from build123d import *

# Parameters (mm, degrees)
SKETCH1_R           = 1.5875
SKETCH1_W           = 12.7
SKETCH1_H           = 6.35
SKETCH1_W_2         = 6.35
BOSS_EXTRUDE1_DEPTH = 6.35


with BuildPart() as part:
    # Sketch1 → Boss-Extrude1 (new body)
    # profile 1 of 6: a face of its own
    with BuildSketch(Plane(origin=(0, 0, 0), x_dir=(1, 0, 0), z_dir=(0, 1, 0))):
        Polygon((355.6, 19.05), (177.8, 19.05), (177.8, 0), (355.6, 0), (355.6, 6.35), (355.6, 12.7), align=None)
        with Locations(Location((196.05625, 9.525, 0), (0, 0, 270))):
            Circle(SKETCH1_R, mode=Mode.SUBTRACT)
        with Locations((298.45, 9.525)):
            Rectangle(SKETCH1_W, SKETCH1_H, mode=Mode.SUBTRACT)
    # profile 2 of 6: a face of its own
    with BuildSketch(Plane(origin=(0, 0, 0), x_dir=(1, 0, 0), z_dir=(0, 1, 0))):
        Polygon((177.8, 0), (177.8, 19.05), (0, 19.05), (0, 12.7), (0, 6.35), (0, 0), align=None)
        with Locations(Location((159.54375, 9.525, 0), (0, 0, 270))):
            Circle(SKETCH1_R, mode=Mode.SUBTRACT)
    # profile 3 of 6: a face of its own
    with BuildSketch(Plane(origin=(0, 0, 0), x_dir=(1, 0, 0), z_dir=(0, 1, 0))):
        with Locations((-3.175, 15.875)):
            Rectangle(SKETCH1_W_2, SKETCH1_H)
    # profile 4 of 6: a face of its own
    with BuildSketch(Plane(origin=(0, 0, 0), x_dir=(1, 0, 0), z_dir=(0, 1, 0))):
        with Locations((358.775, 15.875)):
            Rectangle(SKETCH1_W_2, SKETCH1_H)
    # profile 5 of 6: a face of its own
    with BuildSketch(Plane(origin=(0, 0, 0), x_dir=(1, 0, 0), z_dir=(0, 1, 0))):
        with Locations((-3.175, 3.175)):
            Rectangle(SKETCH1_W_2, SKETCH1_H)
    # profile 6 of 6: a face of its own
    with BuildSketch(Plane(origin=(0, 0, 0), x_dir=(1, 0, 0), z_dir=(0, 1, 0))):
        with Locations((358.775, 3.175)):
            Rectangle(SKETCH1_W_2, SKETCH1_H)
    extrude(amount=BOSS_EXTRUDE1_DEPTH)


solid = part.part
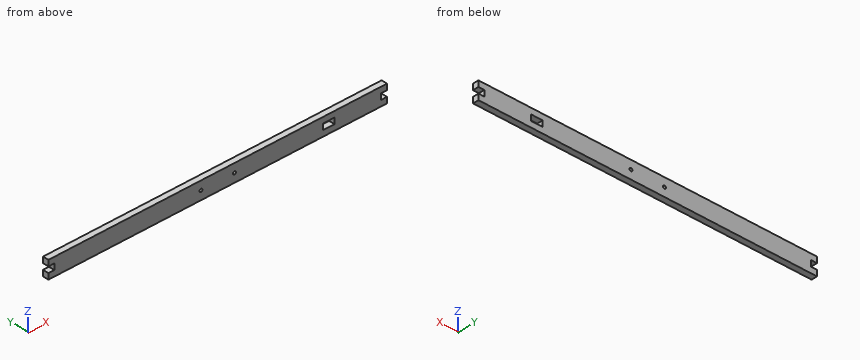
Read the model definition and answer for the solid it produces. Units are mm, in the model's axes. Round coordinates to 2 decimals unless told otherwise and drop trailing zeros. One line per question, with ' | ' between items. Start each with the question number.
1. Find the intervals of material crossed by probe 1 along X at (y, z) = (2.25, -7); probe 2 along X at (y, z) = (6.25, -9); probe 3 along X at (y, z) = (3, -10.25), in increasing order. Write a range as [from, to].
2. This flat-tipped pin is pushed along its axis until it touches: pin 1 (3 mm diameter, centred on y = 3, z = -10, fed in from +X). Where does it stop, or does it pass through?
3. Section A-A (y = 2.25) is taken. Give the number of separate pieces and of enclosed holes in the cut face, and give its area (3 significant figures).
Filled in:
1) probe 1: [0, 292.1], [304.8, 355.6] | probe 2: [0, 158.05], [161.04, 194.56], [197.55, 292.1], [304.8, 355.6] | probe 3: [0, 158.13], [160.96, 194.64], [197.47, 292.1], [304.8, 355.6]
2) pin 1: x = 355.6
3) separate pieces: 1 | enclosed holes: 3 | area: 6,840 mm²
